The drawing under review shows one solid part. Ordinate dimensions are in mm from its lowest x, y, z. A direction names the side the tool comes from. Round coordinates to 2 decimals unless told otherwise and drop trailing zeros. Order: outer loops, then holes, each group sorted by start corner. A loop starts at its lowest first (then second) coordinate and runs counter-clockwise, first axis right, second up. Notation, with made-up numbers: (67.25, 20.5) - (71.25, 20.5) arc R10 ccw to (71.25, 29.5) - close; hole circle Ø9 at (49.5, 37.25). An arc over 180 degrees is marked (long way). Answer as a JSON object with one key per item and string values. Group by question number.
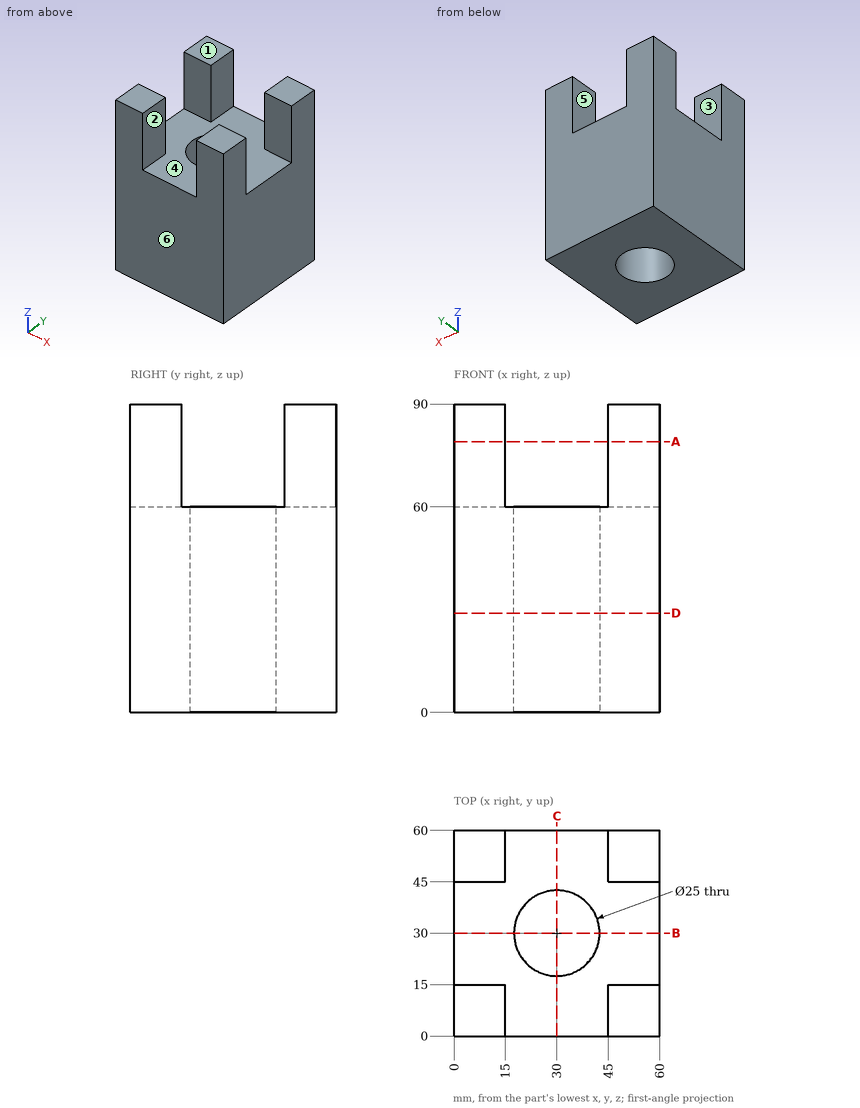
1. Tool access review of the marked faces 1, 2 and 3: name each direction out of +Z, -Z, +X, -X, +Y, -Y from which nothing blocks a thin tool from reaching the whole face with its end or side.
2. Take a section at D-D, the plane z = 29. Give the boundary of the cut face in (x, y).
3. Take a section at A-A, the plane z = 79. Give the boundary of the cut face in (x, y), then the cut area to 3 significant figures.
4. To check wall thickness, follow line 1 (Y direction, x = 30, z = 22); line 2 (Y direction, x = 53.5, z = 68). State the ranges of each line that lie inside material, in increasing order. Write a range as from..to.
5. Mouldability with a two-part tool opening along Y and no side actions: class the marked faces 4, 5 and 6 as pulls with the +Y half, pulls with the -Y half, needs draft (parallel to the pull), parting line crosses it, or undercut.
6. Take a section at B-B, the plane y = 30. Give the boundary of the cut face in (x, z).
7. Clearance check with flat-ended pins moving along their axes: P1, Ø3, axis at x = 46.5, y = 28.5, coming from the -Z side; P2, Ø5, axis at x = 52.5, y = 27, coming from the +Z side. State where each tip first meets the part, or that it passes through.
Response values:
{
 "1": {"face 1": "+Z, +X, -X, +Y, -Y", "face 2": "+Z, +Y, -Y", "face 3": "+Z, +X, -X"},
 "2": {"outline": "(0, 0) - (60, 0) - (60, 60) - (0, 60) - close; hole circle Ø25 at (30, 30)"},
 "3": {"outline": "(0, 0) - (15, 0) - (15, 15) - (0, 15) - close; (0, 45) - (15, 45) - (15, 60) - (0, 60) - close; (45, 0) - (60, 0) - (60, 15) - (45, 15) - close; (45, 45) - (60, 45) - (60, 60) - (45, 60) - close", "area": "900 mm2"},
 "4": {"line 1": "0..17.5, 42.5..60", "line 2": "0..15, 45..60"},
 "5": {"face 4": "undercut", "face 5": "needs draft", "face 6": "pulls with the -Y half"},
 "6": {"outline": "(0, 0) - (17.5, 0) - (17.5, 60) - (0, 60) - close; (42.5, 0) - (60, 0) - (60, 60) - (42.5, 60) - close"},
 "7": {"P1": "z = 0", "P2": "z = 60"}
}
